```python
from build123d import *


with BuildPart() as part:
    # Esquisse1 → Base-Révolution (revolve)
    with BuildSketch(Plane.XY, mode=Mode.PRIVATE) as base_r_volution_sk:
        with BuildLine():
            Line((-15.29638585, 26), (-3.89638585, 26))
            ThreePointArc((-3.89638585, 26), (-3.472121782, 25.824264069), (-3.29638585, 25.4))
            Line((-3.29638585, 25.4), (-3.29638585, 24.811004735))
            ThreePointArc((-3.29638585, 24.811004735), (-3.405550409, 24.465924209), (-3.693321081, 24.246412227))
            Line((-3.693321081, 24.246412227), (-15.493321081, 20.002352589))
            ThreePointArc((-15.493321081, 20.002352589), (-16.041466376, 20.076109655), (-16.29638585, 20.566945096))
            Line((-16.29638585, 20.566945096), (-16.29638585, 25))
            ThreePointArc((-16.29638585, 25), (-16.003492631, 25.707106781), (-15.29638585, 26))
        make_face()
    revolve(base_r_volution_sk.sketch.rotate(Axis((-17.990056753, 0, 0), (1, 0, 0)), 90), axis=Axis((-17.990056753, 0, 0), (1, 0, 0)))


solid = part.part
```
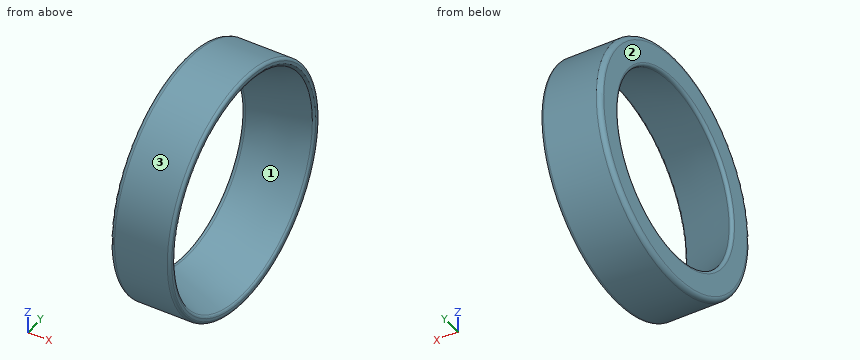
Could you check a few things on this model? Use its own coordinates, in mm. Face numbers are marked on the shaded views. Give positions to 0.01 mm unless a question says otherwise; leave off trailing zeros. Order: outer loops, then holes, each group sorted by start corner. A loop starts at its lowest first (then second) coordinate and runs counter-clockwise, first axis right, second up.
Q1. Suppose I cut it at A-A, the plane z = 0. Write out the boundary of the cut face in (x, y).
Q2. We'd pull the mould along Z, two halves only. Please class the marked faces 1, 2 and 3: +Z half, -Z half, draft (parallel to the pull), parting line (faces both ways), or undercut.
Q3. Suppose I cut it at D-D, the plane x = -5. Write out the boundary of the cut face in (y, z), and give its area (3 significant figures).
Q4. If I drill on line 1 along Z through (x, y) = (-10, 3); line 2 along Y through (x, z) = (-10.5, 2.5); line 3 along Z through (x, y) = (-8, -16), over which ranges is the centre line in solid material (lowest first)?
Q5. Suppose I cut it at C-C, the plane x = -10. Write out the boundary of the cut face in (y, z).
Q6. I'm going to push flat-ended pins straight in: P1, Ø2, axis at x = -14.5, z = -10.5, coming from the -Y side; P2, Ø1, axis at x = -13, z = -10.5, coming from the -Y side; P3, Ø3, axis at x = -11.5, z = -8, coming from the -Y side; P4, Ø12, axis at y = 7, z = 17.5, coming from the -X side. Where does each tip first touch, or does it pass through?
Solution:
1. outline: (-16.3, -25) arc R1 ccw to (-15.3, -26) - (-3.9, -26) arc R0.6 ccw to (-3.3, -25.4) - (-3.3, -24.81) arc R0.6 ccw to (-3.69, -24.25) - (-15.49, -20) arc R0.6 ccw to (-16.3, -20.57) - close; (-16.3, 20.57) arc R0.6 ccw to (-15.49, 20) - (-3.69, 24.25) arc R0.6 ccw to (-3.3, 24.81) - (-3.3, 25.4) arc R0.6 ccw to (-3.9, 26) - (-15.3, 26) arc R1 ccw to (-16.3, 25) - close
2. face 1: undercut
2. face 2: draft
2. face 3: parting line
3. outline: circle Ø52 at (0, 0); hole circle Ø47.55 at (0, 0)
3. area: 348 mm2
4. line 1: z = -25.83 to -21.77, 21.77 to 25.83
4. line 2: y = -25.88 to -21.65, 21.65 to 25.88
4. line 3: z = -20.49 to -16.1, 16.1 to 20.49
5. outline: circle Ø52 at (0, 0); hole circle Ø43.96 at (0, 0)
6. P1: stops at y = -24.2
6. P2: stops at y = -24
6. P3: stops at y = -25.17
6. P4: stops at x = -16.3
